```python
from build123d import *

# Parameters (mm, degrees)
ESQUISSE1_W        = 90
ESQUISSE1_H        = 90
BOSS_EXTRU_1_DEPTH = 20
ESQUISSE5_W        = 110
ESQUISSE5_H        = 90
BOSS_EXTRU_5_DEPTH = 20
ESQUISSE2_R        = 6
BOSS_EXTRU_2_DEPTH = 277
ESQUISSE3_W        = 80
ESQUISSE3_H        = 80
BOSS_EXTRU_3_DEPTH = 2.9
ESQUISSE4_W        = 80
ESQUISSE4_H        = 80
BOSS_EXTRU_4_DEPTH = 0.1


with BuildPart() as part:
    # Esquisse1 → Boss.-Extru.1 (new body)
    with BuildSketch(Plane(origin=(0, 0, 0), x_dir=(0, 0, -1), z_dir=(1, 0, 0))):
        with Locations((30.929303344, -12.964038863)):
            Rectangle(ESQUISSE1_W, ESQUISSE1_H)
    extrude(amount=BOSS_EXTRU_1_DEPTH)

    # Esquisse5 → Boss.-Extru.5 (add)
    with BuildSketch(Plane.XY.offset(14.070696656)):
        with Locations((55, -12.964038863)):
            Rectangle(ESQUISSE5_W, ESQUISSE5_H)
    extrude(amount=BOSS_EXTRU_5_DEPTH)

    # Esquisse2 → Boss.-Extru.2 (add)
    with BuildSketch(Plane(origin=(0, 32.035961137, 0), x_dir=(1, 0, 0), z_dir=(0, 1, 0))):
        with Locations(Location((10, -24.070696656, 0), (0, 0, 90))):
            Circle(ESQUISSE2_R)
    extrude(amount=BOSS_EXTRU_2_DEPTH)

    # Esquisse3 → Boss.-Extru.3 (add)
    with BuildSketch(Plane(origin=(0, 309.035961137, 0), x_dir=(1, 0, 0), z_dir=(0, 1, 0))):
        with Locations((-20, -54.070696656)):
            Rectangle(ESQUISSE3_W, ESQUISSE3_H)
    extrude(amount=BOSS_EXTRU_3_DEPTH)

    # Esquisse4 → Boss.-Extru.4 (add)
    with BuildSketch(Plane(origin=(0, 311.935961137, 0), x_dir=(1, 0, 0), z_dir=(0, 1, 0))):
        with Locations((-20, -54.070696656)):
            Rectangle(ESQUISSE4_W, ESQUISSE4_H)
    extrude(amount=BOSS_EXTRU_4_DEPTH)


solid = part.part
```
Geometry check sheet. Reference: the model listing, model coordinates, mm. A direction names the side the tool comes from. Coordinates: 2 decimals unless noted, no trailing zeros. Write each loop counter-clockwise with the first axis right and the second up, starting at its lowest first coordinate (ties: lowest second). Pieces come first, ordered by that corner, then holes. Notation, with made-up numbers: M -18.5,89.25 L 1.5,89.25 A33 cw 1.5,125.25 Z; hole C 9,-1.5 d9. An arc over 180 degrees is marked long. One line per item, written item: value. Start each with the question number.
(1) Depth check by flat-ended pin: pin 1 (12 mm diameter, centred on x = -2, z = 50.5, fed in from -Y); pin 2 (12 mm diameter, centred on x = 20.5, z = -46, fed in from +Y); pin 3 (8 mm diameter, centred on x = 5.5, y = 220.5, fed in from -Z). Enter the tip coordinate at first touch or a pass-through.
(2) Sectioned sample at D-D, the plane x = 92.5. Enter the section's corners in (y, z), and give its area (3 significant figures).
(3) Sectioned sample at B-B, the plane y = 58.5. Enter the section's corners in (x, z).
(4) Tool access check on faces 4 (the face through (-21, 312.036, 54)), 5 (the face through (0, -14, -22)), 6 (the face through (10, -14, -75.929)), 7 (the face through (64, -12, 14.071)), 8 (the face through (54, -12, 34.071)). Record the directions out of +Z, -Z, +X, -X, +Y, -Y that give a thin tool (end or side, any length) a straight path to the whole face; none if there is none.
(5) Release check for a two-part mould opening along Y. For faces 1 (the face through (18, -57.964, 3)), 2 (the face through (110, -14, 24)), 3 (the face through (8.198, 168.597, 18.348)) record: released by +Y, released by -Y, zero draft, split by the parting line, or undercut.
(6) Sectioned sample at C-C, the plane z = 71. Enter the section's corners in (x, y), and give its area (3 significant figures).
(7) Sectioned sample at A-A, the plane x = 10. Enter the section's corners in (y, z).
(8) Scan lines: line 1 along Z through (x, y) = (38.5, -5); line 2 along Y through (x, z) = (11.5, -23.5); line 3 along Z through (x, y) = (13, 26). Record each from-to range of solid material in increasing order. Write a range as [from, to].
Filled sheet:
1. pin 1: y = 309.04
1. pin 2: y = 32.04
1. pin 3: z = 18.09
2. outline: M -57.96,14.07 L 32.04,14.07 L 32.04,34.07 L -57.96,34.07 Z
2. area: 1,800 mm²
3. outline: C 10,24.07 d12
4. face 4: +Z, -Z, +X, -X, +Y
4. face 5: +Z, -Z, -X, -Y
4. face 6: -Z, +X, -X, +Y, -Y
4. face 7: -Z, +X, +Y, -Y
4. face 8: +Z, +X, -X, -Y
5. face 1: released by -Y
5. face 2: zero draft
5. face 3: undercut
6. outline: M -60,309.04 L 20,309.04 L 20,312.04 L -60,312.04 Z
6. area: 240 mm²
7. outline: M -57.96,-75.93 L 32.04,-75.93 L 32.04,18.07 L 309.04,18.07 L 309.04,14.07 L 312.04,14.07 L 312.04,94.07 L 309.04,94.07 L 309.04,30.07 L 32.04,30.07 L 32.04,34.07 L -57.96,34.07 Z
8. line 1: [14.07, 34.07]
8. line 2: [-57.96, 32.04]
8. line 3: [-75.93, 34.07]
